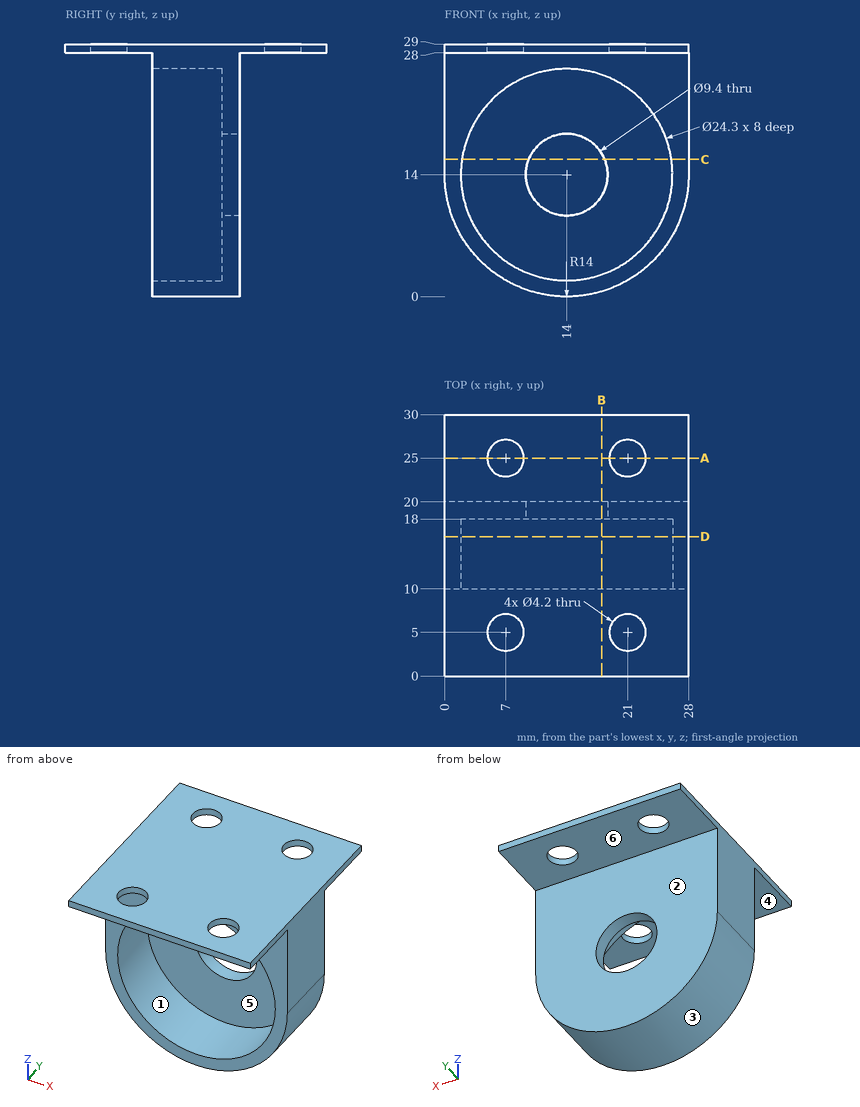
Input: dimensioned drawing with shaded views. Units: mm. Origin: part minimum x, y, z. A direction names the side the tool comes from. Give positions to 0.01 mm unless a question says otherwise; leave off trailing zeros. Write each loop counter-clockwise with the first axis right and the second up, starting at its lowest first coordinate (ties: lowest second). Pieces come first, ordered by that corner, then holes. Notation, with made-up numbers: (86.25, -6) -> (127.25, -6) arc R22 cw to (127.25, 6) -> close; hole circle Ø6 at (15, -24). An arc over 180 degrees is marked (long way). Return JSON: item names as keys, results as strings. Group by question number.
1. Section C-C, the plane z = 15.75. Output: boundary loops of the cut face in (x, y).
2. Access query for the marked faces 4, 5 and 6. Directions: +Z, -Z, +X, -X, +Y, -Y. A direction counts if a zero-diameter tool reaches every point of the face in a straight line with its end or side. Return the directions, or none.
3. Section D-D, the plane y = 16. Output: boundary loops of the cut face in (x, z).
4. Section B-B, the plane x = 18. Output: boundary loops of the cut face in (y, z), then the cut area to 3 significant figures.
5. Mould query, pull axis X, two halves, no side actions, for the marked faces 1, 2 and 3. Classes: +X half, -X half, draft (parallel to the pull), parting line (faces both ways), or undercut.
6. Section A-A, the plane y = 25. Output: boundary loops of the cut face in (x, z).
7. Pin query (flat end, axial travel): pin 1 Ø3 at (x, y) = (15, 6.5) entering from -Z; pin 2 Ø14 at (x, z) = (11, 9) entering from +Y; pin 3 Ø4 at (x, y) = (4.5, 20) entering from -Z. Return the tip coordinate at first contact, or that it passes through.
8. Material intervals for line 1 (Y direction, x = 21, z = 28.25); line 2 (X direction, y = 19.45, z = 14); line 3 (Y direction, x = 8.75, z = 18), sorted ascending. Write a range as from..to.
Determined:
{
 "1": {"outline": "(0, 10) -> (1.98, 10) -> (1.98, 18) -> (9.64, 18) -> (9.64, 20) -> (0, 20) -> close; (18.36, 18) -> (26.02, 18) -> (26.02, 10) -> (28, 10) -> (28, 20) -> (18.36, 20) -> close"},
 "2": {"face 4": "-Z, +X, -X, -Y", "face 5": "-Y", "face 6": "-Z, +X, -X, +Y"},
 "3": {"outline": "(0, 14) arc R14 ccw to (28, 14) -> (28, 29) -> (0, 29) -> close; hole circle Ø24.3 at (14, 14)"},
 "4": {"outline": "(0, 28) -> (10, 28) -> (10, 25.47) -> (18, 25.47) -> (18, 16.47) -> (20, 16.47) -> (20, 28) -> (30, 28) -> (30, 29) -> (0, 29) -> close; (10, 0.58) -> (20, 0.58) -> (20, 11.53) -> (18, 11.53) -> (18, 2.53) -> (10, 2.53) -> close", "area": "111 mm2"},
 "5": {"face 1": "undercut", "face 2": "draft", "face 3": "parting line"},
 "6": {"outline": "(0, 28) -> (4.9, 28) -> (4.9, 29) -> (0, 29) -> close; (9.1, 28) -> (18.9, 28) -> (18.9, 29) -> (9.1, 29) -> close; (23.1, 28) -> (28, 28) -> (28, 29) -> (23.1, 29) -> close"},
 "7": {"pin 1": "stops at z = 28", "pin 2": "stops at y = 20", "pin 3": "stops at z = 2.18"},
 "8": {"line 1": "y = 0..2.9, 7.1..22.9, 27.1..30", "line 2": "x = 0..9.3, 18.7..28", "line 3": "y = 18..20"}
}
